Study the drawing (mm; zero at the part's minimum x, y, z) and answer. Round coordinates to 2 decimals unless told otherwise and drop trailing zeros. Order: outer loops, then holes, each group sorted by start corner. A loop starts at its lowest first (then second) coordinate and runs counter-clockwise, first axis right, second up. Notation, with made-up numbers: (13, -38.75) - (25, -38.75) arc R25 cw to (25, -8.75) - close; hole circle Ø4 at (26.25, 32.5). An arc over 180 degrees is marked (long way). Put each result on its own line as item: value.
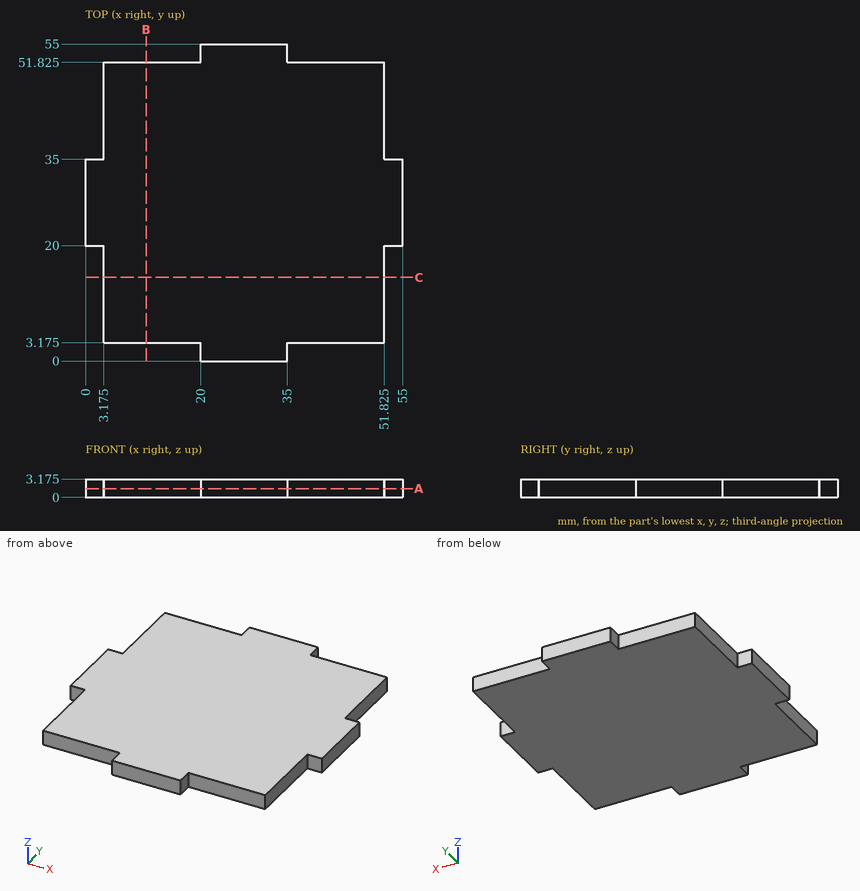
1) A cutting plane is placed at B-B on x = 10.5. Write down the section's boundary in (y, z) (3 decimals), then the cut area to 3 significant figures.
Findings below:
outline: (3.175, 0) - (51.825, 0) - (51.825, 3.175) - (3.175, 3.175) - close
area: 154 mm2
2) A cutting plane is placed at A-A on z = 1.5. Write down the section's boundary in (x, y) (3 decimals).
Findings below:
outline: (0, 20) - (3.175, 20) - (3.175, 3.175) - (20, 3.175) - (20, 0) - (35, 0) - (35, 3.175) - (51.825, 3.175) - (51.825, 20) - (55, 20) - (55, 35) - (51.825, 35) - (51.825, 51.825) - (35, 51.825) - (35, 55) - (20, 55) - (20, 51.825) - (3.175, 51.825) - (3.175, 35) - (0, 35) - close
3) Given pin 1 Ø1.6 at (y, z) = (53.5, 1) entering from +X; pin 2 Ø1 at (y, z) = (10, 2) entering from +X (3 decimals); pin 3 Ø1 at (x, z) = (10.5, 1) entering from -Y (3 decimals), each flat-ended and moving along its own axis, determine where each tip first touches the part or whether it passes through.
Findings below:
pin 1: stops at x = 35
pin 2: stops at x = 51.825
pin 3: stops at y = 3.175
4) Straight lines are drawn through the part: L1, parallel to Y at x = 46.5, z = 1.55 (3 decimals); L2, parallel to X at y = 2.5, z = 2.15. For each, find the intervals that lie inside material, in ascending order. Write a range as from..to.
Findings below:
L1: y = 3.175..51.825
L2: x = 20..35
